from build123d import *

# Parameters (mm, degrees)
F0_W     = 60
F0_H     = 40
F1_DEPTH = 10
F2_W     = 60
F2_H     = 20
F3_DEPTH = 10
F5_DEPTH = 20
F6_R     = 10
F8_DEPTH = 20


with BuildPart() as f1:
    # F0 (on Top) → F1 (new body)
    with BuildSketch(Plane.XY):
        Rectangle(F0_W, F0_H)
    extrude(amount=F1_DEPTH)

    # F2 (on face) → F3 (join)
    with BuildSketch(Plane.XY.offset(10)):
        with Locations((0, -10)):
            Rectangle(F2_W, F2_H)
    extrude(amount=F3_DEPTH)

    # F4 (on face) → F5 (join)
    with BuildSketch(Plane(origin=(0, 0, 0), x_dir=(-1, 0, 0), z_dir=(0, 1, 0))):
        with BuildLine():
            Line((-30, 20), (10, 20))
            ThreePointArc((10, 20), (-10, 40), (-30, 20))
        make_face()
    extrude(amount=-F5_DEPTH)

    # F6
    f6_edges = [f1.edges().sort_by_distance(p)[0] for p in [
        (-30, -10, 20),
    ]]
    fillet(f6_edges, radius=F6_R)

    # F7 (on face) → F8 (cut)
    with BuildSketch(Plane(origin=(0, 0, 0), x_dir=(-1, 0, 0), z_dir=(0, 1, 0))):
        with BuildLine():
            ThreePointArc((-10, 10), (-2.928932, 12.928932), (0, 20))
            ThreePointArc((0, 20), (-17.071068, 27.071068), (-10, 10))
        make_face()
    extrude(amount=-F8_DEPTH, mode=Mode.SUBTRACT)


solid = f1.part
Could you check a few things on this model? Use its own coordinates, in mm. A direction names the side the tool comes from. Give positions to 0.01 mm unless a question says otherwise; leave off trailing zeros. Write each loop counter-clockwise with the first axis right and the second up, starting at its lowest first coordinate (ties: lowest second). Pieces come first, ordered by that corner, then holes. Notation, with made-up numbers: (37.5, 27.25) - (74.5, 27.25) arc R11 ccw to (74.5, 47.25) - close; hole circle Ø11 at (1, 29). An arc over 180 degrees is marked (long way). Use CSV: the item, a comma, the result in double quotes. Start each with the question number.
Item 1: I want a section at B-B, the plane z = 18. Please give me the cut outline in (x, y), then the cut area to 3 significant figures.
Item 2: If I drill on line 1 along Z through (x, y) = (10, -10.5); line 2 along Z through (x, y) = (-9.5, 5.5); line 3 along Y through (x, z) = (25, 15), over which ranges is the centre line in solid material (lowest first)?
Item 3: I'm going to push flat-ended pins straight in: pin 1 (6 mm diameter, centred on x = 10.5, y = 14, fed in from +Z); pin 2 (1 mm diameter, centred on x = -20, y = -14, fed in from +Z); pin 3 (9 mm diameter, centred on x = 8.5, z = 28, fed in from +Y). Where does each tip first touch, or does it pass through?
Item 4: I want a section at D-D, the plane y = 3. Please give me the cut outline in (x, z).
Item 5: For faces 1 (the face through (-15, -10, 20)), 2 (the face through (0, 0, 25)), 3 (the face through (0, 20, 5)), which set-ups out of +Z, -Z, +X, -X, +Y, -Y let a thin tool reach every point of the face, with its end or its side?
Item 6: I want a section at C-C, the plane x = 11. Please give me the cut outline in (y, z), then the cut area to 3 significant figures.
Item 7: I want a section at A-A, the plane y = -14.5. Please give me the cut outline in (x, z).
Findings:
1,outline,"(-26, -20) - (0.2, -20) - (0.2, 0) - (-26, 0) - close; (19.8, -20) - (30, -20) - (30, 0) - (19.8, 0) - close"
1,area,"728 mm2"
2,line 1,"z = 0 to 10, 30 to 40"
2,line 2,"z = 0 to 10"
2,line 3,"y = -20 to 0"
3,pin 1,"stops at z = 10"
3,pin 2,"stops at z = 20"
3,pin 3,"stops at y = 0"
4,outline,"(-30, 0) - (30, 0) - (30, 10) - (-30, 10) - close"
5,face 1,"+Z, -X, +Y, -Y"
5,face 2,"+Z, +X, -X, +Y"
5,face 3,"+Z, -Z, +X, -X, +Y"
6,outline,"(-20, 0) - (20, 0) - (20, 10) - (0, 10) - (0, 10.05) - (-20, 10.05) - close; (-20, 29.95) - (0, 29.95) - (0, 39.97) - (-20, 39.97) - close"
6,area,"602 mm2"
7,outline,"(-30, 0) - (30, 0) - (30, 20) arc R20 ccw to (-10, 20) - (-20, 20) arc R10 ccw to (-30, 10) - close; hole circle Ø20 at (10, 20)"
